from build123d import *

# Parameters (mm, degrees)
SKETCH1_W           = 22
SKETCH1_H           = 28
BOSS_EXTRUDE1_DEPTH = 8
SKETCH2_R           = 2
CUT_EXTRUDE1_DEPTH  = 37.249137921
SKETCH5_R           = 7
SKETCH5_R_2         = 2
BOSS_EXTRUDE3_DEPTH = 5.5


with BuildPart() as part:
    # Sketch1 → Boss-Extrude1 (new body)
    with BuildSketch(Plane(origin=(0, 0, 0), x_dir=(1, 0, 0), z_dir=(0, 1, 0))):
        with BuildLine():
            ThreePointArc((-18, 11), (-13.050252532, 13.050252532), (-11, 18))
            Line((-11, 18), (-18, 18))
            Line((-18, 18), (-18, 11))
        make_face()
        with BuildLine():
            Line((-18, 18), (-11, 18))
            ThreePointArc((-11, 18), (-22.949747468, 22.949747468), (-18, 11))
            Line((-18, 11), (-18, 18))
        make_face()
        with BuildLine():
            Line((-11, -18), (-11, -14))
            Line((-11, -14), (-11, 14))
            Line((-11, 14), (-11, 18))
            ThreePointArc((-11, 18), (-13.050252532, 13.050252532), (-18, 11))
            Line((-18, 11), (-18, -11))
            ThreePointArc((-18, -11), (-13.050252532, -13.050252532), (-11, -18))
        make_face()
        with BuildLine():
            ThreePointArc((-18, -11), (-22.949747468, -22.949747468), (-11, -18))
            Line((-11, -18), (-18, -18))
            Line((-18, -18), (-18, -11))
        make_face()
        with BuildLine():
            Line((-18, -18), (-11, -18))
            ThreePointArc((-11, -18), (-13.050252532, -13.050252532), (-18, -11))
            Line((-18, -11), (-18, -18))
        make_face()
        Rectangle(SKETCH1_W, SKETCH1_H)
        with BuildLine():
            ThreePointArc((18, -11), (13.050252532, -13.050252532), (11, -18))
            Line((11, -18), (18, -18))
            Line((18, -18), (18, -11))
        make_face()
        with BuildLine():
            Line((18, -18), (11, -18))
            ThreePointArc((11, -18), (18, -25), (25, -18))
            ThreePointArc((25, -18), (22.949747468, -13.050252532), (18, -11))
            Line((18, -11), (18, -18))
        make_face()
        with BuildLine():
            Line((11, 14), (11, -14))
            Line((11, -14), (11, -18))
            ThreePointArc((11, -18), (13.050252532, -13.050252532), (18, -11))
            Line((18, -11), (18, 11))
            ThreePointArc((18, 11), (13.050252532, 13.050252532), (11, 18))
            Line((11, 18), (11, 14))
        make_face()
        with BuildLine():
            ThreePointArc((25, 18), (18, 25), (11, 18))
            Line((11, 18), (18, 18))
            Line((18, 18), (18, 11))
            ThreePointArc((18, 11), (22.949747468, 13.050252532), (25, 18))
        make_face()
        with BuildLine():
            Line((18, 18), (11, 18))
            ThreePointArc((11, 18), (13.050252532, 13.050252532), (18, 11))
            Line((18, 11), (18, 18))
        make_face()
    extrude(amount=BOSS_EXTRUDE1_DEPTH)

    # Sketch2 → Cut-Extrude1 (cut, through all)
    with BuildSketch(Plane(origin=(0, 8, 0), x_dir=(1, 0, 0), z_dir=(0, 1, 0))):
        with Locations(Location((-18, 18, 0), (0, 0, 270))):
            Circle(SKETCH2_R)
        with Locations(Location((-18, -18, 0), (0, 0, 270))):
            Circle(SKETCH2_R)
        with Locations(Location((18, -18, 0), (0, 0, 270))):
            Circle(SKETCH2_R)
        with Locations(Location((18, 18, 0), (0, 0, 270))):
            Circle(SKETCH2_R)
    extrude(amount=-CUT_EXTRUDE1_DEPTH, mode=Mode.SUBTRACT)

    # Sketch5 → Boss-Extrude3 (add)
    # profile 1 of 4: a face of its own
    with BuildSketch(Plane.XZ):
        with Locations(Location((-18, 18, 0), (0, 0, 270))):
            Circle(SKETCH5_R)
        with Locations(Location((-18, 18, 0), (0, 0, 90))):
            Circle(SKETCH5_R_2, mode=Mode.SUBTRACT)
    # profile 2 of 4: a face of its own
    with BuildSketch(Plane.XZ):
        with Locations(Location((18, 18, 0), (0, 0, 270))):
            Circle(SKETCH5_R)
        with Locations(Location((18, 18, 0), (0, 0, 90))):
            Circle(SKETCH5_R_2, mode=Mode.SUBTRACT)
    # profile 3 of 4: a face of its own
    with BuildSketch(Plane.XZ):
        with Locations(Location((18, -18, 0), (0, 0, 270))):
            Circle(SKETCH5_R)
        with Locations(Location((18, -18, 0), (0, 0, 90))):
            Circle(SKETCH5_R_2, mode=Mode.SUBTRACT)
    # profile 4 of 4: a face of its own
    with BuildSketch(Plane.XZ):
        with Locations(Location((-18, -18, 0), (0, 0, 270))):
            Circle(SKETCH5_R)
        with Locations(Location((-18, -18, 0), (0, 0, 90))):
            Circle(SKETCH5_R_2, mode=Mode.SUBTRACT)
    extrude(amount=BOSS_EXTRUDE3_DEPTH)


solid = part.part
Could you check a few things on this model? Use its own coordinates, in mm. A direction names the side the tool comes from. Round coordinates to 2 decimals unless told otherwise and drop trailing zeros. Order: outer loops, then holes, each group sorted by start corner. A loop starts at its lowest first (then second) coordinate and runs counter-clockwise, first axis right, second up.
Q1. Imagine slicing it at A-A, the plane y = -1. List the corners of the cut face in (x, z) for me, then the cut area to 3 significant figures.
Geometry says:
outline: circle Ø14 at (-18, -18); circle Ø14 at (-18, 18); circle Ø14 at (18, -18); circle Ø14 at (18, 18); hole circle Ø4 at (-18, -18); hole circle Ø4 at (-18, 18); hole circle Ø4 at (18, -18); hole circle Ø4 at (18, 18)
area: 565 mm2
Q2. Imagine slicing it at C-C, the plane z = 21. List the corners of the cut face in (x, y) for me, then the cut area to 3 significant figures.
Geometry says:
outline: (-24.32, -5.5) - (-11.68, -5.5) - (-11.68, 8) - (-24.32, 8) - close; (11.68, -5.5) - (24.32, -5.5) - (24.32, 8) - (11.68, 8) - close
area: 342 mm2
Q3. Imagine slicing it at D-D, the plane y = 2.25. List the corners of the cut face in (x, z) for me.
Geometry says:
outline: (-18, -11) arc R7 ccw (long way) to (-11, -18) - (-11, -14) - (11, -14) - (11, -18) arc R7 ccw (long way) to (18, -11) - (18, 11) arc R7 ccw (long way) to (11, 18) - (11, 14) - (-11, 14) - (-11, 18) arc R7 ccw (long way) to (-18, 11) - close; hole circle Ø4 at (-18, -18); hole circle Ø4 at (-18, 18); hole circle Ø4 at (18, -18); hole circle Ø4 at (18, 18)
Q4. I'm going to push flat-ended pins straight in: P1, Ø2.5, axis at x = -4.5, y = 5, coming from the +Z side; P2, Ø3, axis at y = 2, z = 15.5, coming from the +X side; P3, Ø4.5, axis at y = 4, z = -15.5, coming from the -X side; P4, Ø4.5, axis at x = -18, z = 18, coming from the +Y side. Where does each tip first touch, or does it pass through?
Geometry says:
P1: stops at z = 14
P2: stops at x = 24.93
P3: stops at x = -25
P4: stops at y = 8
Q5. Thinking about a two-plate mould opening in Z: for faces 1 (the face through (0, 4, -14)), 2 (the face through (11, 4, 16)), 3 (the face through (-18, 4, 0)), 4 (the face through (0, 0, 0)), which applies, released by +Z, released by -Z, zero draft, split by the parting line, or undercut?
Geometry says:
face 1: released by -Z
face 2: zero draft
face 3: undercut
face 4: undercut
Q6. Imagine slicing it at B-B, the plane x = 19. List the corners of the cut face in (y, z) for me, then the cut area to 3 significant figures.
Geometry says:
outline: (-5.5, -24.93) - (8, -24.93) - (8, -19.73) - (-5.5, -19.73) - close; (-5.5, -16.27) - (8, -16.27) - (8, -11.07) - (-5.5, -11.07) - close; (-5.5, 11.07) - (8, 11.07) - (8, 16.27) - (-5.5, 16.27) - close; (-5.5, 19.73) - (8, 19.73) - (8, 24.93) - (-5.5, 24.93) - close
area: 281 mm2
Q7. Please list where these lines run through material, in increasing order: probe 1 along X at (y, z) = (5.75, -18); probe 2 along Y at (x, z) = (-8.5, -7.5).
Geometry says:
probe 1: x = -25 to -20, -16 to -11, 11 to 16, 20 to 25
probe 2: y = 0 to 8
Q8. Which directions (+Z, -Z, +X, -X, +Y, -Y) give clear straight access to the entire face, cutting with the end or side of a thin tool? Please do faces 5 (the face through (0, 8, 0)), 6 (the face through (0, 4, 14)), 7 (the face through (11, 4, -16)), 8 (the face through (20, -5.5, 17)), 9 (the face through (18, 4, 0)).
Geometry says:
face 5: +Z, -Z, +X, -X, +Y
face 6: +Z, +Y, -Y
face 7: -Z, +Y, -Y
face 8: +Z, -Z, +X, -X, -Y
face 9: +X, +Y, -Y
